from build123d import *

# Parameters (mm, degrees)
F0_W     = 177.8
F0_H     = 101.6
F1_DEPTH = 25.4
F2_R     = 57.15
F2_R_2   = 50.8
F3_DEPTH = 50.8
F4_DEPTH = 25.4
F6_DEPTH = 25.4
F8_DEPTH = 25.4


with BuildPart() as f1:
    # F0 (on Top) → F1 (new body)
    with BuildSketch(Plane.XY):
        Rectangle(F0_W, F0_H)
    extrude(amount=F1_DEPTH)

    # F2 (on Top) → F3 (join)
    with BuildSketch(Plane.XY):
        with Locations((101.6, 0)):
            Circle(F2_R)
        with Locations((101.6, 0)):
            Circle(F2_R_2, mode=Mode.SUBTRACT)
    extrude(amount=F3_DEPTH)

    # F2 (on Top) + F3_face (on face) → F4 (cut)
    with BuildSketch(Plane.XY):
        with Locations((101.6, 0)):
            Circle(F2_R)
        with Locations((101.6, 0)):
            Circle(F2_R_2, mode=Mode.SUBTRACT)
    with BuildSketch(Plane(origin=(73.0309989911, 0, 25.4), x_dir=(1, 0, 0), z_dir=(0, 0, 1))):
        with BuildLine():
            ThreePointArc((15.8690010089, 49.1868884968), (-22.2309989911, 0), (15.8690010089, -49.1868884968))
            Line((15.8690010089, -49.1868884968), (15.8690010089, 49.1868884968))
        make_face()
    extrude(amount=-F4_DEPTH, mode=Mode.SUBTRACT)

    # F5 (on face) → F6 (join)
    with BuildSketch(Plane.XY.offset(25.4)):
        with BuildLine():
            Line((0, 11.9811560377), (0, -13.4188439623))
            Line((0, -13.4188439623), (45.72, -13.4188439623))
            Line((45.72, -13.4188439623), (45.72, -11.9811560377))
            ThreePointArc((45.72, -11.9811560377), (44.45, 0), (45.72, 11.9811560377))
            Line((45.72, 11.9811560377), (0, 11.9811560377))
        make_face()
    extrude(amount=F6_DEPTH)

    # F7 (on face) → F8 (cut)
    with BuildSketch(Plane.XZ.offset(13.4188439623)):
        Polygon((0, 25.4), (45.72, 50.8), (0, 50.8), align=None)
    extrude(amount=-F8_DEPTH, mode=Mode.SUBTRACT)


solid = f1.part
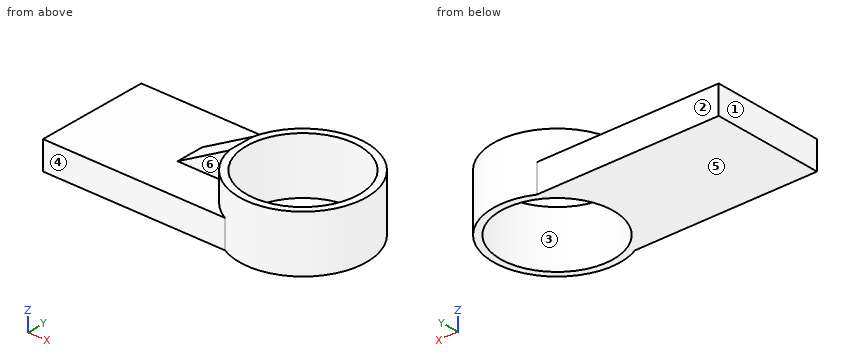
Could you check a few things on this model? Use its own coordinates, in mm. Face numbers are marked on the shaded views. A direction names the side the tool comes from. Give positions to 0.01 mm unless a question says otherwise; leave off trailing zeros. Order: outer loops, then holes, each group sorted by start corner. A loop starts at its lowest first (then second) coordinate and runs counter-clockwise, first axis right, second up. Notation, with made-up numbers: M 19.5,21 L 36.5,21 A21 cw 36.5,57 Z; hole C 11,48 d1. An arc over 180 degrees is marked long. One line per question, with ' | ' between items.
1. I want a section at A-A (x = 101.6). List the corners of the cut face in (y, z) for me, and give its area (3 significant figures).
Results:
outline: M -57.15,0 L -50.8,0 L -50.8,50.8 L -57.15,50.8 Z; M 50.8,0 L 57.15,0 L 57.15,50.8 L 50.8,50.8 Z | area: 645 mm²
2. I want a section at D-D (z = 17.5). List the corners of the cut face in (x, y) for me, and give its area (3 significant figures).
Results:
outline: M -88.9,-50.8 L 75.42,-50.8 A57.15 ccw long 75.42,50.8 L -88.9,50.8 Z; hole C 101.6,0 d101.6 | area: 16,600 mm²
3. I want a section at B-B (y = 0). List the corners of the cut face in (x, z) for me.
Results:
outline: M -88.9,0 L 50.8,0 L 50.8,50.8 L 45.72,50.8 L 0,25.4 L -88.9,25.4 Z; M 152.4,0 L 158.75,0 L 158.75,50.8 L 152.4,50.8 Z
4. If I drill on line 1 (Y direction, x = 101, z = 18); line 2 (Z direction, x = -55, y = 17); line 3 (X direction, y = 9.5, z = 45.5), over which ranges is the centre line in solid material (lowest first)?
Results:
line 1: -57.15 to -50.8, 50.8 to 57.15 | line 2: 0 to 25.4 | line 3: 36.18 to 51.7, 151.5 to 157.95
5. I'm going to push flat-ended pins straight in: pin 1 (6 mm diameter, centred on x = 81.5, z = 20, fed in from +Y); pin 2 (2 mm diameter, centred on x = 128, z = 26.5, fed in from -Y); pin 3 (1.5 mm diameter, centred on x = 70.5, z = 10.5, fed in from -Y). Where does each tip first touch, or does it pass through?
Results:
pin 1: y = 54.53 | pin 2: y = -51.2 | pin 3: y = -50.8
6. For the marked faces 4, 5 and 6, which set-ups out of +Z, -Z, +X, -X, +Y, -Y let a thin tool reach every point of the face, with its end or its side?
Results:
face 4: +Z, -Z, -X, -Y | face 5: -Z, +X, -X, +Y, -Y | face 6: +Z, -X, -Y
7. I want a section at C-C (z = 40). List the corners of the cut face in (x, y) for me, and give its area (3 significant figures).
Results:
outline: M 26.28,-13.42 L 45.72,-13.42 L 45.72,-11.98 A57.15 ccw long 45.72,11.98 L 26.28,11.98 Z; hole C 101.6,0 d101.6 | area: 2,630 mm²
8. We'd pull the mould along Y, two halves only. Please class the marked faces 1, 2 and 3: +Y half, -Y half, draft (parallel to the pull), parting line (faces both ways), or undercut.
Results:
face 1: draft | face 2: +Y half | face 3: undercut
